Autodesk Fusion 360 part; units mm, degrees
sketch "Sketch1" plane through (0, 0, 0) normal (0, 0, 1) x (1, 0, 0)
  line L0 (0, 0) -> (60, 0)
  line L1 (60, 0) -> (60, 20)
  line L2 (60, 20) -> (0, 20)
  line L3 (0, 20) -> (0, 0)
  dimension "d1" = 60
  dimension "d2" = 20
extrude "Extrude1" add sketch "Sketch1" along normal blind 40
sketch "Sketch2" plane through (0, 0, 0) normal (-1, 0, 0) x (0, -1, 0)
  line L0 (-20, 0) -> (0, 0)
  line L1 (0, 0) -> (0, 40)
  line L2 (0, 40) -> (-20, 40)
  line L3 (-20, 40) -> (-20, 0)
  line L4 (-15, 28) -> (-5, 28)
  line L5 (-5, 28) -> (-5, 16)
  line L6 (-5, 16) -> (-15, 16)
  line L7 (-15, 16) -> (-15, 28)
  dimension "d5" = 10
  dimension "d6" = 12
  dimension "d7" = 5
extrude "Extrude2" cut sketch "Sketch2" against normal blind 30 contours L4 L5 L6 L7
extrude "Extrude3" cut 1 faces at (20, 13.3333, 40) along direction (0, 0, -1) blind 2
extrude "Extrude4" cut 1 faces at (20, 13.3333, 0) along direction (0, 0, 1) blind 2
sketch "Sketch3" plane through (0, 20, 0) normal (0, 1, 0) x (-1, 0, 0)
  line L0 (-60, 2) -> (0, 2)
  line L1 (0, 2) -> (0, 38)
  line L2 (0, 38) -> (-60, 38)
  line L3 (-60, 38) -> (-60, 2)
  line L4 (-40, 33) -> (-20, 33)
  line L5 (-20, 33) -> (-20, -1)
  line L6 (-20, -1) -> (-40, -1)
  line L7 (-40, -1) -> (-40, 33)
  dimension "d14" = 20
  dimension "d15" = 34
  dimension "d16" = 20
  dimension "d17" = 5
extrude "Extrude5" cut 1 faces at (20, 13.3333, 2) along direction (0, 0, 1) blind 9
extrude "Extrude6" cut 1 faces at (20, 13.3333, 11) along direction (0, 0, 1) blind 1
extrude "Extrude7" cut sketch "Sketch3" against normal blind 20 contours L0 L4 L5 L7
extrude "Extrude8" cut sketch "Sketch2" against normal blind 80 contours L4 L5 L6 L7
extrude "Extrude9" cut 1 faces at (20, 13.3333, 38) along direction (0, 0, -1) blind 1
extrude "Extrude10" cut 1 faces at (60, 8.3333, 34) along direction (-1, 0, 0) blind 10
extrude "Extrude11" add 1 faces at (40, 1.6667, 24.3333) along direction (-1, 0, 0) blind 10
extrude "Extrude12" cut 1 faces at (50, 8.3333, 34) along direction (-1, 0, 0) blind 10
extrude "Extrude13" cut 1 faces at (6.6667, 20, 27.3333) along direction (0, -1, 0) blind 2
extrude "Extrude14" cut 1 faces at (6.6667, 0, 27.3333) along direction (0, 1, 0) blind 2
extrude "Extrude15" cut 1 faces at (36.6667, 12.6667, 12) along direction (0, 0, 1) blind 1
extrude "Extrude16" cut 1 faces at (13.3333, 7.3333, 12) along direction (0, 0, 1) blind 1
extrude "Extrude17" cut 1 faces at (36.6667, 12.6667, 13) along direction (0, 0, 1) blind 1
extrude "Extrude18" cut 1 faces at (13.3333, 7.3333, 13) along direction (0, 0, 1) blind 1
extrude "Extrude19" cut sketch "Sketch2" against normal blind 2
extrude "Extrude20" cut 1 faces at (14.6667, 7.3333, 37) along direction (0, 0, -1) blind 1
extrude "Extrude21" add 1 faces at (26.6667, 12.6667, 33) along direction (0, 0, -1) blind 1
extrude "Extrude22" cut 1 faces at (14.6667, 7.3333, 36) along direction (0, 0, -1) blind 1
fillet "Fillet1" radius 1 2 faces at (36.6667, 12.6667, 14) (14, 7.3333, 14)
sketch "Sketch4" plane through (2, 0, 0) normal (-1, 0, 0) x (0, -1, 0)
  line L0 (-5, 16) -> (-15, 16)
  line L1 (-15, 16) -> (-15, 28)
  line L2 (-15, 28) -> (-5, 28)
  line L3 (-5, 28) -> (-5, 16)
  line L4 (-18, 15) -> (-2, 15)
  line L5 (-2, 15) -> (-2, 35)
  line L6 (-2, 35) -> (-18, 35)
  line L7 (-18, 35) -> (-18, 15)
  line L8 (-15.5, 28.5) -> (-4.5, 28.5)
  line L9 (-4.5, 28.5) -> (-4.5, 15.5)
  line L10 (-4.5, 15.5) -> (-15.5, 15.5)
  line L11 (-15.5, 15.5) -> (-15.5, 28.5)
  dimension "d56" = 11
  dimension "d57" = 13
  dimension "d58" = 2.5
  dimension "d59" = 6.5
extrude "Extrude23" cut sketch "Sketch4" against normal blind 50 contours L8 L9 L10 L11
extrude "Extrude24" add 2 faces at (36.6667, 8.1667, 15.5) (14, 11.8333, 15.5) along direction (0, 0, 1) blind 1
extrude "Extrude25" cut 2 faces at (33.3333, 11.8333, 28.5) (14, 11.8333, 28.5) along direction (0, 0, 1) blind 1
extrude "Extrude26" cut 1 faces at (26.6667, 12.6667, 32) along direction (0, 0, 1) blind 0.5
Check sheet for the modelled part. Datum: model origin and axes. Units: mm. A direction names the side the tool comes from. Coordinates: 2 decimals unless noted, no trailing zeros. Loops run counter-clockwise (first coordinate to the right, second up) from the corner with the lowest first, then second, coordinate; pieces in that order, holes last. Notation, with made-up numbers: (6, 46.5) -> (28, 46.5) arc R6 ccw to (28, 50.5) -> close; hole circle Ø5 at (30.25, 89). An arc over 180 degrees is marked (long way). Answer in a Markdown table with one row per item.
1. Sectioned sample at C-C, the plane z = 31. Record the boundary of the cut face in (x, y), then the cut area to 3 significant figures.
Check values:
| item | result |
|---|---|
| outline | (2, 2) -> (20, 2) -> (20, 18) -> (2, 18) -> close; (30, 2) -> (40, 2) -> (40, 18) -> (30, 18) -> close |
| area | 448 mm2 |
2. Go/stop test with flat-tipped pins: pin 1 (5 mm diameter, centred on y = 12, z = 21.5, fed in from -X); pin 2 (6 mm diameter, centred on x = 27.5, z = 27, fed in from +Y). Record where each tip stops, or that it passes through.
Check values:
| item | result |
|---|---|
| pin 1 | passes through |
| pin 2 | stops at y = 18 |
3. Access from +Z, -Z, +X, -X, +Y, -Y to the whole of each face (thin tool, end or side, straight path). Record for faces 1 (the face through (21, 10, 35)), 2 (the face through (35, 15.5, 23)), 3 (the face through (30.285, 9.888, 14.301)).
Check values:
| item | result |
|---|---|
| face 1 | +Z, +X, -X, +Y, -Y |
| face 2 | +X, -X |
| face 3 | -Z, +Y, -Y |
4. Sectioned sample at B-B, the plane y = 7.75. Record the boundary of the cut face in (x, z), then the cut area to 3 significant figures.
Check values:
| item | result |
|---|---|
| outline | (2, 15) arc R1 ccw to (3, 14) -> (19, 14) arc R1 ccw to (20, 15) -> (20, 16.5) -> (2, 16.5) -> close; (2, 29.5) -> (20, 29.5) -> (20, 32.5) -> (30, 32.5) -> (30, 29.5) -> (40, 29.5) -> (40, 35) -> (2, 35) -> close; (30, 15) arc R1 ccw to (31, 14) -> (39, 14) arc R1 ccw to (40, 15) -> (40, 16.5) -> (30, 16.5) -> close |
| area | 248 mm2 |
5. Material ranges on line 1 along Y through (x, z) = (36.5, 21.5); line 2 along X through (y, z) = (16, 20.5); line 3 along Z through (x, y) = (38.5, 7), recorded low to high. Write a range as [from, to].
Check values:
| item | result |
|---|---|
| line 1 | y = [2, 4.5], [15.5, 18] |
| line 2 | x = [2, 20], [30, 40] |
| line 3 | z = [14, 16.5], [29.5, 35] |
6. Release check for a two-part mould opening along X. For faces 4 (the face through (19.715, 10.112, 14.301)), 5 (the face through (39.715, 10.112, 14.301)), 6 (the face through (25, 10, 32.5)), 7 (the face through (34.93, 17.715, 14.301)) record: released by +X, released by -X, zero draft, split by the parting line, or undercut.
Check values:
| item | result |
|---|---|
| face 4 | undercut |
| face 5 | released by +X |
| face 6 | undercut |
| face 7 | zero draft |
7. Sectioned sample at A-A, the plane x = 17. Record the boundary of the cut face in (y, z), then the cut area to 3 significant figures.
Check values:
| item | result |
|---|---|
| outline | (2, 15) arc R1 ccw to (3, 14) -> (17, 14) arc R1 ccw to (18, 15) -> (18, 35) -> (2, 35) -> close; hole (4.5, 16.5) -> (15.5, 16.5) -> (15.5, 29.5) -> (4.5, 29.5) -> close |
| area | 193 mm2 |
8. Sectioned sample at D-D, the plane z = 21.75. Record the boundary of the cut face in (x, y), then the cut area to 3 significant figures.
Check values:
| item | result |
|---|---|
| outline | (2, 2) -> (20, 2) -> (20, 4.5) -> (2, 4.5) -> close; (2, 15.5) -> (20, 15.5) -> (20, 18) -> (2, 18) -> close; (30, 2) -> (40, 2) -> (40, 4.5) -> (30, 4.5) -> close; (30, 15.5) -> (40, 15.5) -> (40, 18) -> (30, 18) -> close |
| area | 140 mm2 |
